Geometry check sheet. Reference: the model listing, model coordinates, mm. A direction names the side the tool comes from. Give positions to 0.01 mm unless a question says otherwise; leave off trailing zeros. Loops run counter-clockwise (first coordinate to the right, second up) from the corner with the lowest first, then second, coordinate; pieces in that order, holes last. Notation, with made-up numbers: (82.5, -35.75) -> (119.5, -35.75) arc R25 cw to (119.5, -14.75) -> close; hole circle Ø9 at (82, 9.25). An arc over 180 degrees is marked (long way). Answer as a JSON object with one key per item and string values.
from build123d import *

# Parameters (mm, degrees)
SKETCH1_W           = 94.5
SKETCH1_H           = 70
BOSS_EXTRUDE1_DEPTH = 3
SKETCH2_R           = 14
SKETCH2_R_2         = 1.5
SKETCH2_W           = 3.5
SKETCH2_H           = 21
CUT_EXTRUDE1_DEPTH  = 59.877521177
FILLET1_R           = 0.5
SKETCH3_R           = 1.5
CUT_EXTRUDE2_DEPTH  = 59.877521177
FILLET2_R           = 3


with BuildPart() as part:
    # Sketch1 → Boss-Extrude1 (new body)
    with BuildSketch(Plane(origin=(0, 0, 0), x_dir=(1, 0, 0), z_dir=(0, 1, 0))):
        Rectangle(SKETCH1_W, SKETCH1_H)
    extrude(amount=BOSS_EXTRUDE1_DEPTH)

    # Sketch2 → Cut-Extrude1 (cut, through all)
    with BuildSketch(Plane(origin=(0, 3, 0), x_dir=(1, 0, 0), z_dir=(0, 1, 0))):
        with Locations(Location((-17.25, -0.5, 0), (0, 0, 270))):
            Circle(SKETCH2_R)
        with Locations(Location((-5.25, 11.5, 0), (0, 0, 270))):
            Circle(SKETCH2_R_2)
        with Locations(Location((-29.25, 11.5, 0), (0, 0, 270))):
            Circle(SKETCH2_R_2)
        with Locations(Location((-29.25, -12.5, 0), (0, 0, 270))):
            Circle(SKETCH2_R_2)
        with Locations(Location((-5.25, -12.5, 0), (0, 0, 270))):
            Circle(SKETCH2_R_2)
        Polygon((-36.25, 25), (23.75, 25), (23.75, 13), (12.75, 13), (12.75, 16), (-36.25, 16), align=None)
        with Locations((-36.5, -4.5)):
            Rectangle(SKETCH2_W, SKETCH2_H)
        with Locations((5.5, -14.5)):
            Rectangle(SKETCH2_W, SKETCH2_H)
    extrude(amount=-CUT_EXTRUDE1_DEPTH, mode=Mode.SUBTRACT)

    # Fillet1
    fillet1_edges = [part.edges().sort_by_distance(p)[0] for p in [
        (3.75, 1.5, 25),
        (3.75, 1.5, 4),
        (7.25, 1.5, 4),
        (7.25, 1.5, 25),
        (-38.25, 1.5, -6),
        (-34.75, 1.5, -6),
        (-34.75, 1.5, 15),
        (-38.25, 1.5, 15),
        (-36.25, 1.5, -16),
        (-36.25, 1.5, -25),
        (23.75, 1.5, -25),
        (23.75, 1.5, -13),
        (12.75, 1.5, -13),
        (12.75, 1.5, -16),
    ]]
    fillet(fillet1_edges, radius=FILLET1_R)

    # Sketch3 → Cut-Extrude2 (cut, through all)
    with BuildSketch(Plane(origin=(0, 3, 0), x_dir=(1, 0, 0), z_dir=(0, 1, 0))):
        with Locations(Location((43.75, 31.5, 0), (0, 0, 270))):
            Circle(SKETCH3_R)
        with Locations(Location((-43.25, 31.5, 0), (0, 0, 270))):
            Circle(SKETCH3_R)
        with Locations(Location((-43.25, -31.5, 0), (0, 0, 270))):
            Circle(SKETCH3_R)
        with Locations(Location((43.75, -31.5, 0), (0, 0, 270))):
            Circle(SKETCH3_R)
    extrude(amount=-CUT_EXTRUDE2_DEPTH, mode=Mode.SUBTRACT)

    # Fillet2
    fillet2_edges = [part.edges().sort_by_distance(p)[0] for p in [
        (47.25, 1.5, 35),
        (-47.25, 1.5, 35),
        (-47.25, 1.5, -35),
        (47.25, 1.5, -35),
    ]]
    fillet(fillet2_edges, radius=FILLET2_R)


solid = part.part
1) Material ranges on line 1 along X through (y, z) = (1.15, -31.5); line 2 along Z through (x, y) = (6.5, 0.3); line 3 along Z through (x, y) = (-37.5, 1.8), recorded low to high. Write a range as from..to.
Geometry check:
{"line 1": "x = -47.25..-44.75, -41.75..42.25, 45.25..47.25", "line 2": "z = -35..-25, -16..4, 25..35", "line 3": "z = -35..-6, 15..35"}
2) Draft check along Z on faces 1 (the face through (-34.75, 2, 5)), 2 (the face through (5, 2, 4)), 3 (the face through (-1, 1, 35)), 4 (the face through (47.25, 1, 0)). Enter one of: pulls with the +Z half, pulls with the -Z half, needs draft (parallel to the pull), parting line crosses it, or undercut.
Geometry check:
{"face 1": "undercut", "face 2": "undercut", "face 3": "pulls with the +Z half", "face 4": "needs draft"}
3) Section check C-C on x = -5.25. Record the cut outline in (y, z).
Geometry check:
{"outline": "(0, -35) -> (3, -35) -> (3, -25) -> (0, -25) -> close; (0, -16) -> (3, -16) -> (3, -13) -> (0, -13) -> close; (0, -10) -> (3, -10) -> (3, -6.71) -> (0, -6.71) -> close; (0, 7.71) -> (3, 7.71) -> (3, 11) -> (0, 11) -> close; (0, 14) -> (3, 14) -> (3, 35) -> (0, 35) -> close"}
4) Tool access check on faces 5 (the face through (-1, 0, 0)), 6 (the face through (5, 2, 25)). Record the directions out of +Z, -Z, +X, -X, +Y, -Y that give a thin tool (end or side, any length) a straight path to the whole face; none if there is none.
Geometry check:
{"face 5": "+Z, -Z, +X, -X, -Y", "face 6": "+Y, -Y"}
5) Section check D-D on z = 9. Record the cut outline in (x, y), plus the area to 3 significant figures.
Geometry check:
{"outline": "(-47.25, 0) -> (-38.25, 0) -> (-38.25, 3) -> (-47.25, 3) -> close; (-34.75, 0) -> (-28.37, 0) -> (-28.37, 3) -> (-34.75, 3) -> close; (-6.13, 0) -> (3.75, 0) -> (3.75, 3) -> (-6.13, 3) -> close; (7.25, 0) -> (47.25, 0) -> (47.25, 3) -> (7.25, 3) -> close", "area": "196 mm2"}
6) Section check B-B on z = 16. Record the cut outline in (x, y), plus the area to 3 significant figures.
Geometry check:
{"outline": "(-47.25, 0) -> (3.75, 0) -> (3.75, 3) -> (-47.25, 3) -> close; (7.25, 0) -> (47.25, 0) -> (47.25, 3) -> (7.25, 3) -> close", "area": "273 mm2"}
7) Depth check by flat-ended pin: P1, Ø2.5, axis at x = -29.25, z = -11.5, coming from the -Y side; P2, Ø3.5, axis at x = -5.25, z = -11.5, coming from the -Y side. Enter the tip coordinate at first touch or a pass-through.
Geometry check:
{"P1": "passes through", "P2": "stops at y = 0"}
8) Section check A-A on x = 5.5. Record the cut outline in (y, z).
Geometry check:
{"outline": "(0, -35) -> (3, -35) -> (3, -25) -> (0, -25) -> close; (0, -16) -> (3, -16) -> (3, 4) -> (0, 4) -> close; (0, 25) -> (3, 25) -> (3, 35) -> (0, 35) -> close"}
